Geometry check sheet. Reference: the model listing, model coordinates, mm. Coordinates: 2 decimals unless noted, no trailing zeros. Write each loop counter-clockwise with the first axis right and the second up, starting at its lowest first coordinate (ties: lowest second). Pieces come first, ordered by that corner, then holes. Notation, with made-up numbers: (-22, 74) -> (36, 74) arc R23 cw to (36, 104) -> close; hole circle Ø4 at (10, 80). An arc over 180 degrees is marked (long way). Answer as CSV lines item,"result".
Autodesk Inventor part; units mm, degrees
ref_plane "XZ Plane" through (0, 0, 0) normal (0, 1, 0) x (-1, 0, 0)
ref_plane "XY Plane" through (0, 0, 0) normal (0, 0, 1) x (1, 0, 0)
sketch "Sketch1" plane through (0, 0, 0) normal (0, 1, 0) x (-1, 0, 0)
  line L0 (0, 0) -> (60, 0)
  line L1 (60, 0) -> (60, -120)
  line L2 (60, -120) -> (0, -120)
  line L3 (0, -120) -> (0, 0)
  line L4 (60, 0) -> (0, -120) construction
  line L5 (60, -120) -> (0, 0) construction
  circle A0 centre (30, -60) radius 67.082
  line L6 (30, -120) -> (30, 7.082) construction
  line L7 (60, -60) -> (0, -60)
  line L8 (30, -60) -> (81.3878, -103.1195) construction
  circle A1 centre (82.6371, -93.7245) radius 1.5
  circle A2 centre (54.2934, -69.9413) radius 1.5
  line L9 (41.76, -45.985) -> (17.4815, -74.919) construction
  circle A3 centre (72.3525, -105.9812) radius 1.5
  circle A4 centre (44.0088, -82.198) radius 1.5
  line L10 (-33, -36.9566) -> (-33, -83.0434)
  line L11 (93, -36.9566) -> (93, -83.0434)
  circle A5 centre (49.1511, -76.0697) radius 1.5
  circle A6 centre (60, -110) radius 1.5
  circle A7 centre (75, -60) radius 12.5
  circle A8 centre (30, -95) radius 7.5
  circle A9 centre (84.4498, -80.8618) radius 1.5
  circle A10 centre (64.472, -88.9254) radius 7.5
  circle A11 centre (30, -60) radius 12.5
  point P0 (60, -120)
  point P1 (60, 0)
  dimension "d0" = 120
  dimension "d25" = 60
  dimension "d27" = 50
  dimension "d28" = 3
  dimension "d30" = 3
  dimension "d32" = 25
  dimension "d33" = 62
  dimension "d34" = 8
  dimension "d35" = 8
  dimension "d38" = 63
  dimension "d39" = 63
  dimension "d40" = 3
  dimension "d41" = 25
  dimension "d50" = 3
  dimension "d51" = 10
  dimension "d52" = 25
  dimension "d53" = 45
  dimension "d54" = 15
  dimension "d55" = 35
  dimension "d56" = 15
  dimension "d57" = 45
  dimension "d58" = 25
extrude "Extrusion1" add sketch "Sketch1" along normal blind 3 contours L0 L1 L7 A11 L3 | L3 A0 L10 | A0 L11 L1 A6 A10 | L7 A11 L1 A10 A6 L2 L3 | A11 L7 | L7 A11 | A10 L1 | L1 A10 | A6 L1 | L1 A6 | A1 | A2 | A3 | A4 | A5 | A7 | A8 | A9
extrude "Extrusion3" cut sketch "Sketch1" along normal blind 10 contours A11 L7 | L7 A11 | A10 L1 | L1 A10 | A6 L1 | L1 A6 | A1 | A2 | A3 | A4 | A5 | A7 | A8 | A9
ref_plane "Work Plane5" through (-60, 0, -60) normal (0, 0, 1) x (1, 0, 0)
ref_plane "Work Plane6" through (-30, 0, 0) normal (1, 0, 0) x (0, 1, 0)
mirror "Mirror3" about plane through (-60, 0, -60) normal (0, 0, 1) of "Extrusion3"
mirror "Mirror4" about plane through (-30, 0, 0) normal (1, 0, 0) of "Extrusion3", "Mirror3"
sketch "Sketch7" plane through (0, 0, 0) normal (0, -1, 0) x (1, 0, 0)
  circle A0 centre (-25.05, -112) radius 1.5
  circle A1 centre (-34.95, -112) radius 1.5
  line L0 (0, -120) -> (-60, -120)
  line L1 (-30, 28.4216) -> (-30, -148.4216)
  point P0 (0, 0)
  dimension "d42" = 3
  dimension "d43" = 3
  dimension "d44" = 8
  dimension "d45" = 8
  dimension "d46" = 4.95
  dimension "d47" = 4.95
extrude "Extrusion4" cut sketch "Sketch7" against normal blind 100
mirror "Mirror5" about plane through (-60, 0, -60) normal (0, 0, 1) of "Extrusion4"
sketch "Sketch10" plane through (0, 3, 0) normal (0, 1, 0) x (1, 0, 0)
  circle A0 centre (-34.95, 8) radius 1.5
  circle A1 centre (-25.05, 8) radius 1.5
  circle A2 centre (-34.95, 112) radius 1.5
  circle A3 centre (-25.05, 112) radius 1.5
  circle A4 centre (24.4498, 39.1382) radius 1.5
  circle A5 centre (-10.8489, 43.9303) radius 1.5
  circle A6 centre (-5.7066, 50.0587) radius 1.5
  circle A7 centre (12.3525, 14.0188) radius 1.5
  circle A8 centre (4.472, 31.0746) radius 7.5
  circle A9 centre (0, 10) radius 1.5
  circle A10 centre (-15.9912, 37.802) radius 1.5
  circle A11 centre (22.6371, 26.2755) radius 1.5
  circle A12 centre (24.4498, 80.8618) radius 1.5
  circle A13 centre (-10.8489, 76.0697) radius 1.5
  circle A14 centre (-5.7066, 69.9413) radius 1.5
  circle A15 centre (12.3525, 105.9812) radius 1.5
  circle A16 centre (15, 60) radius 12.5
  circle A17 centre (4.472, 88.9254) radius 7.5
  circle A18 centre (0, 110) radius 1.5
  circle A19 centre (-15.9912, 82.198) radius 1.5
  circle A20 centre (22.6371, 93.7245) radius 1.5
  circle A21 centre (-84.4498, 39.1382) radius 1.5
  circle A22 centre (-49.1511, 43.9303) radius 1.5
  circle A23 centre (-54.2934, 50.0587) radius 1.5
  circle A24 centre (-72.3525, 14.0188) radius 1.5
  circle A25 centre (-64.472, 31.0746) radius 7.5
  circle A26 centre (-60, 10) radius 1.5
  circle A27 centre (-44.0088, 37.802) radius 1.5
  circle A28 centre (-82.6371, 26.2755) radius 1.5
  circle A29 centre (-30, 25) radius 7.5
  circle A30 centre (-84.4498, 80.8618) radius 1.5
  circle A31 centre (-49.1511, 76.0697) radius 1.5
  circle A32 centre (-54.2934, 69.9413) radius 1.5
  circle A33 centre (-72.3525, 105.9812) radius 1.5
  circle A34 centre (-75, 60) radius 12.5
  circle A35 centre (-64.472, 88.9254) radius 7.5
  circle A36 centre (-60, 110) radius 1.5
  circle A37 centre (-44.0088, 82.198) radius 1.5
  circle A38 centre (-82.6371, 93.7245) radius 1.5
  circle A39 centre (-30, 95) radius 7.5
  circle A40 centre (-30, 60) radius 12.5
  line L0 (0, 120) -> (-60, 120)
  arc A41 (-60, 120) -> (-93, 83.0434) centre (-30, 60) ccw
  line L1 (-93, 83.0434) -> (-93, 36.9566)
  arc A42 (-93, 36.9566) -> (-60, 0) centre (-30, 60) ccw
  line L2 (-60, 0) -> (0, 0)
  arc A43 (0, 0) -> (33, 36.9566) centre (-30, 60) ccw
  line L3 (33, 36.9566) -> (33, 83.0434)
  arc A44 (33, 83.0434) -> (0, 120) centre (-30, 60) ccw
equation "\"d45\" = d44"
equation "\"d47\" = d46"
properties part number "Drone_plate_1"
Item 1: Cross-section at D-D, the plane y = 2.1. Count the separate pieces of the cut face and the enclosed holes in it, plus the area to 3 significant figures.
Responses:
separate pieces,"1"
enclosed holes,"41"
area,"10,600 mm2"
Item 2: Cross-section at A-A, the plane z = -60. Record the cut outline in (x, y).
Responses:
outline,"(-93, 0) -> (-87.5, 0) -> (-87.5, 3) -> (-93, 3) -> close; (-62.5, 0) -> (-42.5, 0) -> (-42.5, 3) -> (-62.5, 3) -> close; (-17.5, 0) -> (2.5, 0) -> (2.5, 3) -> (-17.5, 3) -> close; (27.5, 0) -> (33, 0) -> (33, 3) -> (27.5, 3) -> close"
Item 3: Thickness scan on probe 1 along Z at (x, y) = (-30, 1.75); probe 2 along Z at (x, y) = (-44, 0.35); probe 3 along X at (y, z) = (1.8, -30). Record the ranges inside material, lowest first.
Responses:
probe 1,"z = -120 to -102.5, -87.5 to -72.5, -47.5 to -32.5, -17.5 to 0"
probe 2,"z = -120 to -83.7, -80.7 to -39.3, -36.3 to 0"
probe 3,"x = -90 to -71.89, -57.05 to -35.59, -24.41 to -2.95, 11.89 to 30"
Item 4: Cross-section at B-B, the plane x = -30. Record the cut outline in (y, z), plus the area to 3 significant figures.
Responses:
outline,"(0, -120) -> (3, -120) -> (3, -102.5) -> (0, -102.5) -> close; (0, -87.5) -> (3, -87.5) -> (3, -72.5) -> (0, -72.5) -> close; (0, -47.5) -> (3, -47.5) -> (3, -32.5) -> (0, -32.5) -> close; (0, -17.5) -> (3, -17.5) -> (3, 0) -> (0, 0) -> close"
area,"195 mm2"
Item 5: Release check for a two-part mould opening along X. For faces 1 (the flat face through (-30, 1, -120)), 2 (the cylindrical face through (-44.7, 1.48, -36.47)), 3 (the cylindrical face through (-80.273, 1.479, -104.414)) record: +X half, -X half, draft (parallel to the pull), parting line (faces both ways), or undercut.
Responses:
face 1,"draft"
face 2,"undercut"
face 3,"-X half"
Item 6: Cross-section at C-C, the plane z = -20. Record the cut outline in (x, y).
Responses:
outline,"(-83.85, 0) -> (-35.59, 0) -> (-35.59, 3) -> (-83.85, 3) -> close; (-24.41, 0) -> (23.85, 0) -> (23.85, 3) -> (-24.41, 3) -> close"
Item 7: Depth check by flat-ended pin: pin 1 Ø5 at (x, z) = (0, -110) entering from +Y. Enter the tip coordinate at first touch or a pass-through.
Responses:
pin 1,"stops at y = 3"
